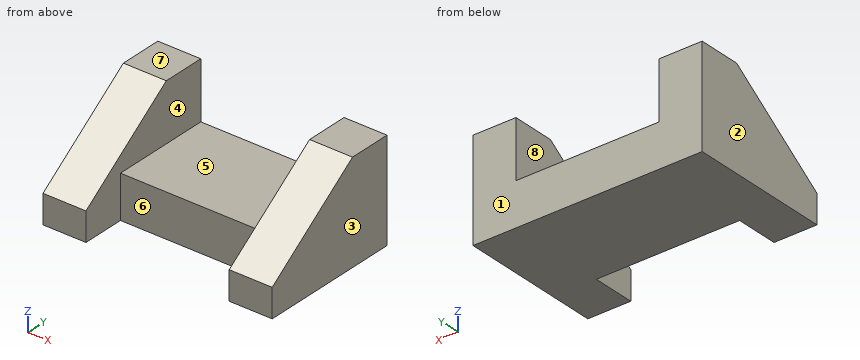
```python
from build123d import *

# Parameters (mm, degrees)
F0_W     = 19.050004
F0_H     = 12.7
F0_W_2   = 19.05
F1_DEPTH = 63.5
F3_W     = 63.5
F3_H     = 19.05
F4_DEPTH = 19.05
F5_DEPTH = 39.99707
F7_DEPTH = 47.63301


with BuildPart() as f1:
    # F0 (on Front) → F1 (new body)
    with BuildSketch(Plane.XZ):
        Polygon((-24.340652, 0), (-24.340652, 25.4), (-43.390656, 25.4), (-43.390656, -6.35), (-24.340652, -6.35), align=None)
        Polygon((39.159348, 0), (-24.340652, 0), (-24.340652, -6.35), (-24.340652, -19.05), (39.159348, -19.05), (39.159348, -6.35), align=None)
        with Locations((-33.865654, -12.7)):
            Rectangle(F0_W, F0_H)
        Polygon((39.159348, 25.4), (39.159348, 0), (39.159348, -6.35), (58.209348, -6.35), (58.209348, 25.4), align=None)
        with Locations((48.684348, -12.7)):
            Rectangle(F0_W_2, F0_H)
    extrude(amount=F1_DEPTH)

    # F3 (on face) → F4 (cut)
    with BuildSketch(Plane.XZ.offset(63.5)):
        with Locations((7.409348, -9.525)):
            Rectangle(F3_W, F3_H)
    extrude(amount=-F4_DEPTH, mode=Mode.SUBTRACT)

    # F2 (on face) → F5 (cut)
    with BuildSketch(Plane.YZ.offset(58.209348)):
        Polygon((-63.5, 25.4), (-63.5, -6.35), (-19.05, 25.4), align=None)
    extrude(amount=-F5_DEPTH, mode=Mode.SUBTRACT)

    # F6 (on face) → F7 (cut)
    with BuildSketch(Plane(origin=(-43.390656, 0, 0), x_dir=(0, -1, 0), z_dir=(-1, 0, 0))):
        Polygon((19.05, 25.4), (63.5, -6.35), (63.5, 25.4), align=None)
    extrude(amount=-F7_DEPTH, mode=Mode.SUBTRACT)


solid = f1.part
```
Geometry: final body of the model. Coordinates: model frame, mm. Face numbers are marked on the shaded views. A direction names the side the tool comes from. Round coordinates to 2 decimals unless told otherwise and drop trailing zeros. Write each loop counter-clockwise with the first axis right and the second up, starting at its lowest first coordinate (ties: lowest second). Pieces come first, ordered by that corner, then holes. Notation, with made-up numbers: (3.25, 12.25) -> (17.25, 12.25) arc R24 cw to (17.25, 23.25) -> close; hole circle Ø4 at (27, -27.75). An arc over 180 degrees is marked (long way). Use CSV: the item, a comma, the result in double quotes. Start each with the question number.
Q1. Section D-D (y = -13). Return loops of the section in (x, z).
Q2. Pull-direction query (X, two-part tool) for the marked faces 1, 2, 3 and 4; classes: pulls with the +X half, pulls with the -X half, needs draft (parallel to the pull), parting line crosses it, or undercut.
Q3. Line query: L1, parallel to X at y = -51.5, z = -8.5; L2, parallel to Z at x = 2, y = -39.5; L3, parallel to Y at x = 33.5, z = -5.5. Output: solid intervals per line, ascending.
Q4. First-contact query: pin 1 Ø5.5 at (x, z) = (-2.5, -13) entering from -Y; pin 2 Ø13.5 at (x, y) = (21, -31.5) entering from +Z; pin 3 Ø1.5 at (x, y) = (38.5, -51.5) entering from -Z; pin 4 Ø12 at (y, z) = (-51.5, 15) entering from -X. Flat tips, straight axial feed; report the tip coordinate or a pass-through.
Q5. Section C-C (z = -14). Return loops of the section in (x, y).
Q6. Reachability of the marked faces 5, 6, 7 and 8 from +Z, -Z, +X, -X, +Y, -Y: full face, straight path, thin tool, end or side. Return the list, or none.
Q7. Section A-A (z = 19). Return loops of the section in (x, y), plus the area to 3 significant figures.
Q8. Section B-B (y = -57.5). Return loops of the section in (x, z).
Result sheet:
1,outline,"(-43.39, -19.05) -> (58.21, -19.05) -> (58.21, 25.4) -> (39.16, 25.4) -> (39.16, 0) -> (-24.34, 0) -> (-24.34, 25.4) -> (-43.39, 25.4) -> close"
2,face 1,"needs draft"
2,face 2,"pulls with the -X half"
2,face 3,"pulls with the +X half"
2,face 4,"undercut"
3,L1,"-43.39 to -24.34, 39.16 to 58.21"
3,L2,"-19.05 to 0"
3,L3,"-44.45 to 0"
4,pin 1,"y = -44.45"
4,pin 2,"z = 0"
4,pin 3,"z = -19.05"
4,pin 4,"through"
5,outline,"(-43.39, -63.5) -> (-24.34, -63.5) -> (-24.34, -44.45) -> (39.16, -44.45) -> (39.16, -63.5) -> (58.21, -63.5) -> (58.21, 0) -> (-43.39, 0) -> close"
6,face 5,"+Z, +Y, -Y"
6,face 6,"+Z, -Z, -Y"
6,face 7,"+Z, +X, -X, +Y, -Y"
6,face 8,"+Z, -Y"
7,outline,"(-43.39, -28.01) -> (-24.34, -28.01) -> (-24.34, 0) -> (-43.39, 0) -> close; (39.16, -28.01) -> (58.21, -28.01) -> (58.21, 0) -> (39.16, 0) -> close"
7,area,"1,070 mm²"
8,outline,"(-43.39, -19.05) -> (-24.34, -19.05) -> (-24.34, -2.06) -> (-43.39, -2.06) -> close; (39.16, -19.05) -> (58.21, -19.05) -> (58.21, -2.06) -> (39.16, -2.06) -> close"
